Model file for the job. Use its own axes, mm. A direction names the side the tool comes from. Round coordinates to 2 decimals unless told otherwise and drop trailing zeros. Order: outer loops, then holes, each group sorted by start corner. A loop starts at its lowest first (then second) coordinate and runs counter-clockwise, first axis right, second up. Notation, with made-up numbers: (10.25, 65) - (24.25, 65) arc R30 cw to (24.25, 94) - close; hole circle Ø3 at (-12.5, 50). An arc over 180 degrees is marked (long way). Write item = value, one per line. Start each with the question number.
from build123d import *

# Parameters (mm, degrees)
BOSS_EXTRUDE1_DEPTH         = 4.7625
F_4_CLEARANCE_HOLE1_D       = 3.4544
F_6_CLEARANCE_HOLE1_D       = 4.3053
F_3_4_0_75_DIAMETER_HOLE1_D = 19.05


with BuildPart() as part:
    # Sketch1 → Boss-Extrude1 (new body)
    with BuildSketch(Plane.XY):
        with BuildLine():
            Line((11.2395, 14.2875), (11.2395, 0.79375))
            Line((11.2395, 0.79375), (134.8105, 0.79375))
            Line((134.8105, 0.79375), (134.8105, 14.2875))
            ThreePointArc((134.8105, 14.2875), (136.670371939, 18.777628061), (141.1605, 20.6375))
            Line((141.1605, 20.6375), (145.25625, 20.6375))
            Line((145.25625, 20.6375), (145.25625, 55.5625))
            Line((145.25625, 55.5625), (141.1605, 55.5625))
            ThreePointArc((141.1605, 55.5625), (136.670371939, 57.422371939), (134.8105, 61.9125))
            Line((134.8105, 61.9125), (134.8105, 75.40625))
            Line((134.8105, 75.40625), (11.2395, 75.40625))
            Line((11.2395, 75.40625), (11.2395, 61.9125))
            ThreePointArc((11.2395, 61.9125), (9.379628061, 57.422371939), (4.8895, 55.5625))
            Line((4.8895, 55.5625), (0.79375, 55.5625))
            Line((0.79375, 55.5625), (0.79375, 20.6375))
            Line((0.79375, 20.6375), (4.8895, 20.6375))
            ThreePointArc((4.8895, 20.6375), (9.379628061, 18.777628061), (11.2395, 14.2875))
        make_face()
    extrude(amount=BOSS_EXTRUDE1_DEPTH)

    # #4 Clearance Hole1 (through all)
    with Locations(Plane.XY.offset(4.7625)):
        with Locations((33.3375, 43.18), (33.3375, 13.97)):
            Hole(F_4_CLEARANCE_HOLE1_D / 2)

    # #6 Clearance Hole1 (through all)
    with Locations(Plane.XY.offset(4.7625)):
        with Locations((34.925, 66.04), (111.125, 66.04), (100.01504, 10.16)):
            Hole(F_6_CLEARANCE_HOLE1_D / 2)

    # 3/4 (0.75) Diameter Hole1 (through all)
    with Locations(Plane.XY.offset(4.7625)):
        with Locations((119.0625, 28.575), (95.25, 45.466), (62.23, 45.466), (33.3375, 28.575)):
            Hole(F_3_4_0_75_DIAMETER_HOLE1_D / 2)


solid = part.part
Item 1: Saw through at B-B, the plane x = 95.25. Give the cut face in (y, z).
Item 2: Probe L1, parallel to Y at x = 62.23, z = 3.45; L2, parallel to Y at x = 63, z = 2.1; L3, parallel to X at y = 40.5, z = 0.35. List the from-to ranges inside material, lowest first.
Item 3: Saw through at D-D, the plane z = 3.8. Give the number of separate pieces and of enclosed holes in the cut face, then the cut area to 3 significant figures.
Item 4: Mould opens along X. For faces 5 (the face through (136.621, 18.728, 2.348)), 6 (the face through (33.93, 64.13, 2.35)), 7 (the face through (72, 39, 0)) say: +X half, -X half, draft (parallel to the pull), parting line (faces both ways), or undercut.
Item 5: Saw through at A-A, the plane y = 66.04. Give the cut face in (x, z).
Item 6: Which spindle directions (+Z, -Z, +X, -X, +Y, -Y) get a long thin tool onto all of the face, cutting with end or side? Do faces 1 (the face through (11.24, 8, 2)), 2 (the face through (11.24, 69, 2)), 3 (the face through (143, 55.562, 2)), 4 (the face through (72, 39, 4.762)). Say none if no direction does.
Item 7: Saw through at C-C, the plane y = 10.16. Give the cut face in (x, z), then the cut area to 3 significant figures.
Item 8: Drop flat-ended pins along their axis: pin 1 (1.4 mm diameter, centred on y = 9, z = 2.5, fed in from +X); pin 2 (2 mm diameter, centred on x = 2, z = 3.5, fed in from +Y); pin 3 (2 mm diameter, centred on x = 3, z = 3, fed in from -Y); pin 4 (4 mm diameter, centred on x = 111.125, y = 66.04, fed in from +Z). Give the stop position or say it passes through.
Check sheet entries:
q1.outline = (0.79, 0) - (35.94, 0) - (35.94, 4.76) - (0.79, 4.76) - close; (54.99, 0) - (75.41, 0) - (75.41, 4.76) - (54.99, 4.76) - close
q2.L1 = 0.79 to 35.94, 54.99 to 75.41
q2.L2 = 0.79 to 35.97, 54.96 to 75.41
q2.L3 = 0.79 to 54.1, 70.36 to 87.12, 103.38 to 145.26
q3.separate_pieces = 1
q3.enclosed_holes = 9
q3.area = 8,780 mm2
q4.face_5 = +X half
q4.face_6 = undercut
q4.face_7 = draft
q5.outline = (11.24, 0) - (32.77, 0) - (32.77, 4.76) - (11.24, 4.76) - close; (37.08, 0) - (108.97, 0) - (108.97, 4.76) - (37.08, 4.76) - close; (113.28, 0) - (134.81, 0) - (134.81, 4.76) - (113.28, 4.76) - close
q6.face_1 = +Z, -Z, -X, -Y
q6.face_2 = +Z, -Z, -X, +Y
q6.face_3 = +Z, -Z, +X, +Y
q6.face_4 = +Z, +X, -X, +Y, -Y
q7.outline = (11.24, 0) - (97.86, 0) - (97.86, 4.76) - (11.24, 4.76) - close; (102.17, 0) - (134.81, 0) - (134.81, 4.76) - (102.17, 4.76) - close
q7.area = 568 mm2
q8.pin_1 = 134.81
q8.pin_2 = 55.56
q8.pin_3 = 20.64
q8.pin_4 = through
